Check sheet for the drawn part. Datum: minimum x, y, z corner. Units: mm. A direction names the side the tool comes from. Coordinates: 2 decimals unless noted, no trailing zeros. Order: outer loops, then holes, each group sorted by start corner. A loop starts at its lowest first (then second) coordinate and runs counter-clockwise, first axis right, second up. Notation, with made-up numbers: (72.5, 43.5) - (118.5, 43.5) arc R7 cw to (118.5, 49.5) - close; hole circle Ø10 at (72.5, 25.5). An arc over 180 degrees is marked (long way). Return JSON: item names as keys, results as strings. Group by question number.
Item 1: Scan lines: probe 1 along Y at (x, z) = (1.5, 0.1); probe 2 along X at (y, z) = (10.75, 1.1); probe 3 along Z at (x, y) = (6.5, 1). Record each from-to range of solid material in increasing order.
Item 2: Section check A-A on y = 3.75. Enter the section's corners in (x, z).
Item 3: Section check D-D on x = 3.5. Enter the section's corners in (y, z).
Item 4: Tool access check on the marked faces 1, 2 and 3. Record the directions out of +Z, -Z, +X, -X, +Y, -Y that give a thin tool (end or side, any length) a straight path to the whole face; none if there is none.
Item 5: Section check C-C on x = 6.35. Enter the section's corners in (y, z).
Item 6: Section check B-B on z = 1.27. Enter the section's corners in (x, y).
Item 7: Draft check along X on the marked faces 4, 5 and 6. Enter one of: pulls with the +X half, pulls with the -X half, needs draft (parallel to the pull), parting line crosses it, or undercut.
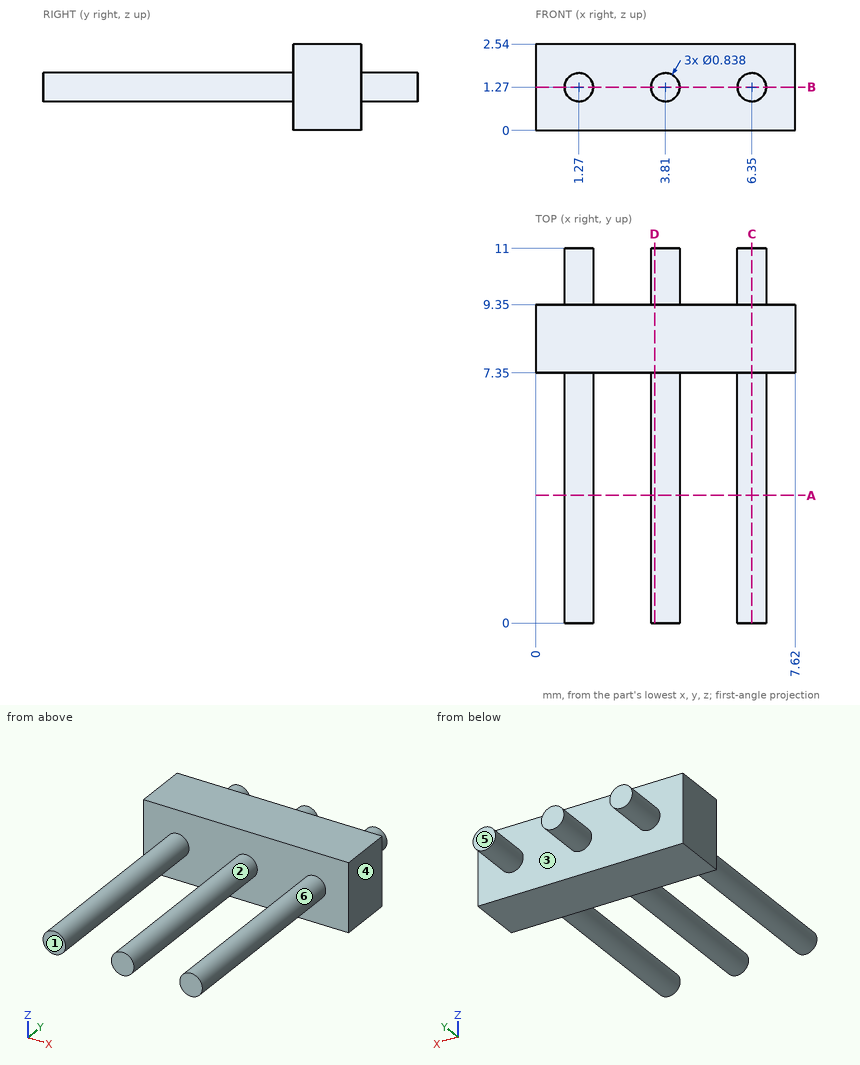
Computed:
{
 "1": {"probe 1": "y = 7.35 to 9.35", "probe 2": "x = 0.89 to 1.65, 3.43 to 4.19, 5.97 to 6.73", "probe 3": "z = 0.88 to 1.66"},
 "2": {"outline": "circle Ø0.84 at (1.27, 1.27); circle Ø0.84 at (3.81, 1.27); circle Ø0.84 at (6.35, 1.27)"},
 "3": {"outline": "(0, 0.99) - (7.35, 0.99) - (7.35, 0) - (9.35, 0) - (9.35, 0.99) - (11, 0.99) - (11, 1.55) - (9.35, 1.55) - (9.35, 2.54) - (7.35, 2.54) - (7.35, 1.55) - (0, 1.55) - close"},
 "4": {"face 1": "+Z, -Z, +X, -X, -Y", "face 2": "-Y", "face 3": "+Y"},
 "5": {"outline": "(0, 0.85) - (7.35, 0.85) - (7.35, 0) - (9.35, 0) - (9.35, 0.85) - (11, 0.85) - (11, 1.69) - (9.35, 1.69) - (9.35, 2.54) - (7.35, 2.54) - (7.35, 1.69) - (0, 1.69) - close"},
 "6": {"outline": "(0, 7.35) - (0.85, 7.35) - (0.85, 0) - (1.69, 0) - (1.69, 7.35) - (3.39, 7.35) - (3.39, 0) - (4.23, 0) - (4.23, 7.35) - (5.93, 7.35) - (5.93, 0) - (6.77, 0) - (6.77, 7.35) - (7.62, 7.35) - (7.62, 9.35) - (6.77, 9.35) - (6.77, 11) - (5.93, 11) - (5.93, 9.35) - (4.23, 9.35) - (4.23, 11) - (3.39, 11) - (3.39, 9.35) - (1.69, 9.35) - (1.69, 11) - (0.85, 11) - (0.85, 9.35) - (0, 9.35) - close"},
 "7": {"face 4": "pulls with the +X half", "face 5": "needs draft", "face 6": "undercut"}
}
